```python
from build123d import *

# Parameters (mm, degrees)
BASE_EXTRUSION_DEPTH     = 315
ESQUISSE3_R              = 1.75
ENL_V_MAT_EXTRU_2_DEPTH  = 3
ENL_V_MAT_EXTRU_5_DEPTH  = 3
ENL_V_MAT_EXTRU_6_DEPTH  = 3
ENL_V_MAT_EXTRU_9_DEPTH  = 3
ESQUISSE8_R              = 3.5
ENL_V_MAT_EXTRU_10_DEPTH = 3
CHANFREIN1_SIZE          = 0.5


with BuildPart() as part:
    # Esquisse1 → Base-Extrusion (new body)
    with BuildSketch(Plane.XY):
        Polygon((0, 0), (0, 25), (25, 25), (25, 22.5), (2.5, 22.5), (2.5, 0), align=None)
    extrude(amount=BASE_EXTRUSION_DEPTH)

    # Esquisse3 → Enlèv. mat.-Extru.2 (cut)
    with BuildSketch(Plane(origin=(0, 25, 0), x_dir=(-1, 0, 0), z_dir=(0, 1, 0))):
        with Locations(Location((-18.3, 61, 0), (0, 0, 90))):
            Circle(ESQUISSE3_R)
        with Locations(Location((-8, 83, 0), (0, 0, 90))):
            Circle(ESQUISSE3_R)
        with Locations(Location((-20, 155, 0), (0, 0, 90))):
            Circle(ESQUISSE3_R)
        with Locations(Location((-8, 230, 0), (0, 0, 90))):
            Circle(ESQUISSE3_R)
        with Locations(Location((-20, 252, 0), (0, 0, 90))):
            Circle(ESQUISSE3_R)
        with Locations(Location((-18.3, 305, 0), (0, 0, 90))):
            Circle(ESQUISSE3_R)
    extrude(amount=-ENL_V_MAT_EXTRU_2_DEPTH, mode=Mode.SUBTRACT)

    # Esquisse5 → Enlèv. mat.-Extru.5 (cut)
    with BuildSketch(Plane(origin=(0, 25, 0), x_dir=(-1, 0, 0), z_dir=(0, 1, 0))):
        Polygon((-3, 0), (-25, 22), (-25, 0), align=None)
    extrude(amount=-ENL_V_MAT_EXTRU_5_DEPTH, mode=Mode.SUBTRACT)

    # Esquisse6 → Enlèv. mat.-Extru.6 (cut)
    with BuildSketch(Plane.ZY):
        Polygon((315, 12), (303, 0), (315, 0), align=None)
    extrude(amount=-ENL_V_MAT_EXTRU_6_DEPTH, mode=Mode.SUBTRACT)

    # Esquisse7 → Enlèv. mat.-Extru.9 (cut)
    with BuildSketch(Plane.ZY):
        with BuildLine():
            Line((255, 0), (255, 13.5))
            ThreePointArc((255, 13.5), (255.732233047, 15.267766953), (257.5, 16))
            Line((257.5, 16), (272.5, 16))
            ThreePointArc((272.5, 16), (274.267766953, 15.267766953), (275, 13.5))
            Line((275, 13.5), (275, 0))
            Line((275, 0), (255, 0))
        make_face()
    extrude(amount=-ENL_V_MAT_EXTRU_9_DEPTH, mode=Mode.SUBTRACT)

    # Esquisse8 → Enlèv. mat.-Extru.10 (cut)
    with BuildSketch(Plane.ZY):
        with Locations((310, 15.5)):
            Circle(ESQUISSE8_R)
        with Locations((5, 15.5)):
            Circle(ESQUISSE8_R)
    extrude(amount=-ENL_V_MAT_EXTRU_10_DEPTH, mode=Mode.SUBTRACT)

    # Chanfrein1
    chanfrein1_edges = [part.edges().sort_by_distance(p)[0] for p in [
        (0, 12.5, 0),
        (0, 0, 127.5),
        (0, 25, 157.5),
        (0, 6.75, 255),
        (0, 18.5, 315),
        (0, 15.267766953, 255.732233047),
        (0, 6, 309),
        (0, 16, 265),
        (0, 0, 289),
        (0, 15.267766953, 274.267766953),
        (0, 6.75, 275),
        (0, 15.5, 306.5),
        (0, 15.5, 1.5),
        (1.5, 25, 0),
        (14, 25, 11),
        (25, 25, 168.5),
        (12.5, 25, 315),
        (8, 25, 228.25),
        (18.3, 25, 303.25),
        (20, 25, 250.25),
        (8, 25, 81.25),
        (20, 25, 153.25),
        (18.3, 25, 59.25),
    ]]
    chamfer(chanfrein1_edges, length=CHANFREIN1_SIZE)


solid = part.part
```
Design review of the part built by this model. Coordinates are the model's own, in mm. A direction names the side the tool comes from. Give positions to 0.01 mm unless a question says otherwise; leave off trailing zeros. Write each loop counter-clockwise with the first axis right and the second up, starting at its lowest first coordinate (ties: lowest second). Pieces come first, ordered by that corner, then holes.
(1) Mouldability with a two-part tool opening along Y and no side actions: class faces 3 (the face through (1.49, 16.55, 8.34)), 4 (the face through (12, 25, 155)), 5 (the face through (0, 12, 155)) as +Y half, -Y half, draft (parallel to the pull), parting line (faces both ways), or undercut.
Checked values:
face 3: undercut
face 4: +Y half
face 5: draft
(2) Clearance check with flat-ended pins moving along their axes: pin 1 Ø6 at (y, z) = (8, 182.5) entering from +X; pin 2 Ø5.5 at (y, z) = (15.5, 5) entering from +X; pin 3 Ø1.6 at (x, y) = (1, 3.5) entering from +Z; pin 4 Ø10 at (x, z) = (12, 100.5) entering from -Y. State where each tip first meets the part, or that it passes through.
Checked values:
pin 1: stops at x = 2.5
pin 2: passes through
pin 3: stops at z = 307.3
pin 4: stops at y = 22.5
(3) Add section A-A (z = 161). Give the boundary of the cut face in (x, y).
Checked values:
outline: (0, 0.5) - (0.5, 0) - (2.5, 0) - (2.5, 22.5) - (25, 22.5) - (25, 24.5) - (24.5, 25) - (0.5, 25) - (0, 24.5) - close
(4) Tool access review of faces 1 (the face through (2.5, 11, 155)), 2 (the face through (1.49, 16.55, 313.34)): name each direction out of +Z, -Z, +X, -X, +Y, -Y from which nothing blocks a thin tool from reaching the whole face with its end or side.
Checked values:
face 1: +Z, -Z, +X, -Y
face 2: +X, -X
(5) Add section B-B (y = 3.5). Give the boundary of the cut face in (x, z), and give its area (3 significant figures).
Checked values:
outline: (0, 0.5) - (0.5, 0) - (2.5, 0) - (2.5, 255) - (0.5, 255) - (0, 254.5) - close; (0, 275.5) - (0.5, 275) - (2.5, 275) - (2.5, 306.5) - (0.5, 306.5) - (0, 305.79) - close
area: 716 mm2
(6) Wall thickness on line 1 along X through (y, z) = (23.45, 83); line 2 along X through (y, z) = (23.6, 155); line 3 along X through (y, z) = (12, 199.5): over which ranges is each line inside the solid? List them lowest first.
Checked values:
line 1: x = 0 to 6.25, 9.75 to 25
line 2: x = 0 to 18.25, 21.75 to 25
line 3: x = 0 to 2.5
